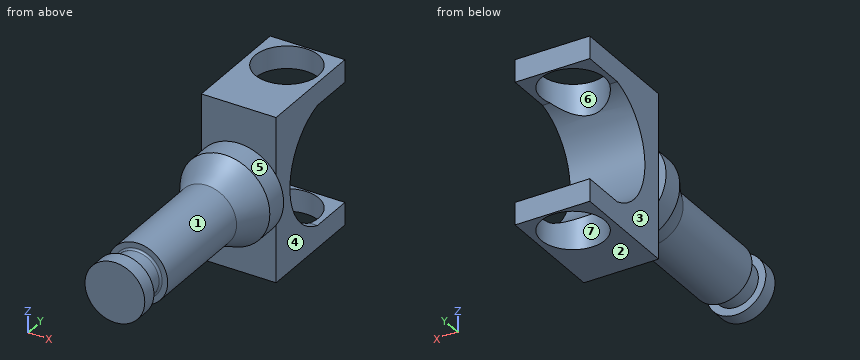
Autodesk Inventor part; units mm, degrees
ref_plane "YZ Plane" through (0, 0, 0) normal (1, 0, 0) x (0, 1, 0)
ref_plane "XZ Plane" through (0, 0, 0) normal (0, 1, 0) x (-1, 0, 0)
ref_plane "XY Plane" through (0, 0, 0) normal (0, 0, 1) x (1, 0, 0)
sketch "Sketch1" plane through (0, 0, 0) normal (0, 0, 1) x (1, 0, 0)
  point P0 (0, 0)
sketch "Sketch2" plane through (0, 0, 0) normal (0, 1, 0) x (-1, 0, 0)
  line L0 (0, 0) -> (0, -22)
  line L1 (0, -22) -> (10, -22)
  line L2 (10, -22) -> (10, 0)
  line L3 (10, 0) -> (0, 0)
  dimension "d0" = 22
  dimension "d1" = 10
extrude "Extrusion1" add sketch "Sketch2" along normal blind 15
sketch "Sketch5" plane through (0, 0, 0) normal (1, 0, 0) x (0, 0, -1)
  line L0 (0, 0) -> (22, 0)
  line L1 (22, 0) -> (22, 15)
  line L2 (0, 15) -> (22, 15)
  line L3 (0, 0) -> (0, 15)
  line L4 (22, 15) -> (0, 15)
  line L5 (0, 15) -> (3, 15)
  line L6 (22, 15) -> (19, 15)
  line L7 (22, 0) -> (0, 0)
  line L8 (11, 0) -> (11, 3)
  line L9 (3, 15) -> (3, 9)
  line L10 (3, 9) -> (19, 9)
  line L11 (19, 9) -> (19, 15)
  arc A0 (3, 9) -> (19, 9) centre (11, 11.3333) ccw
  dimension "d4" = 3
  dimension "d5" = 3
  dimension "d7" = 3
  dimension "d8" = 6
extrude "Extrusion2" cut sketch "Sketch5" against normal blind 17 contours A0 L10 | L2 L11 L10 L9
sketch "Sketch6" plane through (-10, 0, 0) normal (0, 0, 1) x (1, 0, 0)
  line L0 (0, 0) -> (10, 0)
  line L1 (10, 0) -> (10, 15)
  line L2 (0, 15) -> (10, 15)
  line L3 (0, 0) -> (0, 15)
  line L4 (0, 15) -> (10, 15)
  line L5 (5, 15) -> (5, 10.5)
  circle A0 centre (5, 10.5) radius 4.25
  dimension "d11" = 4.5
  dimension "d12" = 8.5
extrude "Extrusion3" cut sketch "Sketch6" against normal blind 31.25 contours A0
sketch "Sketch7" plane through (0, 0, 0) normal (0, -1, 0) x (1, 0, 0)
  line L0 (0, -22) -> (-10, -22)
  line L1 (0, 0) -> (0, -22)
  line L2 (-10, 0) -> (0, 0)
  line L3 (-10, -22) -> (-10, 0)
  line L4 (0, -3) -> (0, -19)
  circle A0 centre (-5, -11) radius 6
  dimension "d15" = 12
extrude "Extrusion4" add sketch "Sketch7" along normal blind 3 contours A0 L3 | L3 A0 L1 | L1 A0
sketch "Sketch8" plane through (-5, -3, -11) normal (0, -1, 0) x (1, 0, 0)
  circle A0 centre (0, 0) radius 6
  circle A1 centre (0, 0) radius 4
  point P0 (5, 11)
  dimension "d18" = 8
extrude "Extrusion5" add sketch "Sketch8" along normal blind 4 contours A1
fillet "Fillet1" radius 28 1 edges at (-9, -3, -11)
sketch "Sketch11" plane through (-5, -7, -11) normal (0, -1, 0) x (1, 0, 0)
  circle A0 centre (0, 0) radius 4
  point P0 (5, 11)
extrude "Extrusion6" add sketch "Sketch11" along normal blind 15
sketch "Sketch12" plane through (-5, -22, -11) normal (0, -1, 0) x (1, 0, 0)
  circle A0 centre (0, 0) radius 3
  point P0 (5, 11)
  dimension "d24" = 6
extrude "Extrusion7" add sketch "Sketch12" along normal blind 3
sketch "Sketch13" plane through (-5, -25, -11) normal (0, -1, 0) x (1, 0, 0)
  circle A0 centre (0, 0) radius 4
  point P0 (5, 11)
extrude "Extrusion8" add sketch "Sketch13" along normal blind 2
fillet "Fillet2" radius 0.25 1 edges at (-8, -22, -11)
Source: CAD feature listing. Evaluate the final solid. Frame: model axes, mm. Face numbers are marked on the shaded views. A direction names the side the tool comes from. Round coordinates to 2 decimals unless told otherwise and drop trailing zeros. Loops run counter-clockwise (first coordinate to the right, second up) from the corner with the lowest first, then second, coordinate; pieces in that order, holes last.
Q1. Section D-D, the plane y = -23. Return loops of the section in (x, z), plus the area to 3 significant figures.
Q2. Access query for the marked faces 1, 2 and 3. Directions: +Z, -Z, +X, -X, +Y, -Y. A direction counts if a zero-diameter tool reaches every point of the face in a straight line with its end or side. Return the directions, or none.
Q3. Mould query, pull axis X, two halves, no side actions, for the marked faces 4, 5, 6 and 7. Classes: pulls with the +X half, pulls with the -X half, needs draft (parallel to the pull), parting line crosses it, or undercut.
Q4. Section B-B, the plane x = -5. State how many separate pieces and enclosed holes the cut face has, plus the area to 3 significant figures.
Q5. Ray query, line 1 (X direction, y = 10.5, z = -2.65); line 2 (Y direction, x = -5, z = -19.7); line 3 (Z direction, x = -9.75, y = 13). Return the intervals inside material, ascending.
Q6. Section A-A, the plane y = 10.5. Return loops of the section in (x, z), plus the area to 3 significant figures.
Q7. First-contact query: P1, Ø4, axis at x = -6.5, z = -13, coming from the +Y side; P2, Ø4, axis at x = -4, z = -19, coming from the -Y side; P3, Ø6, axis at x = -5, y = 0, coming from the +Z side; P4, Ø0.8, axis at x = -10.5, z = -11.5, coming from the +Y side. Flat tips, straight axial feed; report the tip coordinate or a pass-through.
Q8. Section C-C, the plane z = -11. Return loops of the section in (x, y), plus the area to 3 significant figures.
Solutions:
1. outline: circle Ø6 at (-5, -11)
1. area: 28.3 mm2
2. face 1: -Y
2. face 2: -Z, +X, -X, +Y, -Y
2. face 3: +Z, -Z, -X, +Y
3. face 4: pulls with the +X half
3. face 5: parting line crosses it
3. face 6: undercut
3. face 7: undercut
4. separate pieces: 3
4. enclosed holes: 0
4. area: 339 mm2
5. line 1: x = -10 to -9.25, -0.75 to 0
5. line 2: y = 0 to 6.25, 14.75 to 15
5. line 3: z = -22 to -19, -3 to 0
6. outline: (-10, -22) - (-9.25, -22) - (-9.25, -19) - (-10, -19) - close; (-10, -3) - (-9.25, -3) - (-9.25, 0) - (-10, 0) - close; (-0.75, -22) - (0, -22) - (0, -19) - (-0.75, -19) - close; (-0.75, -3) - (0, -3) - (0, 0) - (-0.75, 0) - close
6. area: 9.00 mm2
7. P1: stops at y = 4.02
7. P2: stops at y = 0
7. P3: stops at z = 0
7. P4: stops at y = 0
8. outline: (-11, -3) arc R28 cw to (-9, -7) - (-9, -22) - (-8.25, -22) arc R0.25 cw to (-8, -22.25) - (-8, -25) - (-9, -25) - (-9, -27) - (-1, -27) - (-1, -25) - (-2, -25) - (-2, -22.25) arc R0.25 cw to (-1.75, -22) - (-1, -22) - (-1, -7) arc R28 cw to (1, -3) - (1, 0) - (0, 0) - (0, 3) - (-10, 3) - (-10, 0) - (-11, 0) - close
8. area: 259 mm2
